Source: CAD feature listing. Evaluate the final solid. Frame: model axes, mm. A direction names the side the tool comes from. Round coordinates to 2 decimals unless told otherwise and drop trailing zeros. Loops run counter-clockwise (first coordinate to the right, second up) from the corner with the lowest first, then second, coordinate; pieces in that order, holes last. Notation, with made-up numbers: M 55.25,89.5 L 98.25,89.5 A26 ccw 98.25,111.5 Z; hole C 70,81.25 d9. An arc over 180 degrees is marked long. One line per item, written item: value.
from build123d import *

# Parameters (mm, degrees)
SKETCH1_R                      = 1.27
SKETCH1_R_2                    = 3.81
BOSS_EXTRUDE1_DEPTH            = 5.08
F_15_0_18_DIAMETER_HOLE1_D     = 4.572
SKETCH5_W                      = 15.24
SKETCH5_H                      = 3.81
CUT_EXTRUDE1_DEPTH             = 5.08
FILLET1_R                      = 1.27
CUT_EXTRUDE3_START             = 5.334
SKETCH8_R                      = 1.651
CUT_EXTRUDE3_DEPTH             = 0.762
SCALE1_SCALE                   = 1.5
F_35_0_11_DIAMETER_HOLE1_D     = 2.794
F_35_0_11_DIAMETER_HOLE1_DEPTH = 6.35
F_35_0_11_DIAMETER_HOLE1_TIP   = 0.839402285


with BuildPart() as part:
    # Sketch1 → Boss-Extrude1 (new, symmetric)
    with BuildSketch(Plane.XY):
        with BuildLine():
            Line((-20.909409051, -2.54), (-4.399409051, -2.54))
            ThreePointArc((-4.399409051, -2.54), (5.08, 0), (-4.399409051, 2.54))
            Line((-4.399409051, 2.54), (-20.909409051, 2.54))
            ThreePointArc((-20.909409051, 2.54), (-23.449409051, 0), (-20.909409051, -2.54))
        make_face()
        with Locations((-20.909409051, 0)):
            Circle(SKETCH1_R, mode=Mode.SUBTRACT)
        Circle(SKETCH1_R_2, mode=Mode.SUBTRACT)
    extrude(amount=BOSS_EXTRUDE1_DEPTH, both=True)

    # #15 (0.18) Diameter Hole1 (through all)
    with Locations(Plane(origin=(0, 2.54, 0), x_dir=(1, 0, 0), z_dir=(0, 1, 0))):
        with Locations((-12.019409051, 0)):
            Hole(F_15_0_18_DIAMETER_HOLE1_D / 2)

    # Sketch5 → Cut-Extrude1 (cut)
    with BuildSketch(Plane(origin=(0, 2.54, 0), x_dir=(1, 0, 0), z_dir=(0, 1, 0))):
        with Locations((-23.449409051, 0)):
            Rectangle(SKETCH5_W, SKETCH5_H)
    extrude(amount=-CUT_EXTRUDE1_DEPTH, mode=Mode.SUBTRACT)

    # Fillet1
    fillet1_edges = [part.edges().sort_by_distance(p)[0] for p in [
        (-15.829409051, 0, 1.905),
        (-15.829409051, 0, -1.905),
    ]]
    fillet(fillet1_edges, radius=FILLET1_R)

    # Sketch8 → Cut-Extrude3 (cut)
    with BuildSketch(Plane(origin=(0, 0, 0), x_dir=(0, 0, -1), z_dir=(1, 0, 0)).offset(CUT_EXTRUDE3_START)):
        Circle(SKETCH8_R)
    extrude(amount=-CUT_EXTRUDE3_DEPTH, mode=Mode.SUBTRACT)


with BuildPart() as part_1:
    # Scale1: scaled about (-8.355295552, 4.7607e-05, -6.308e-06)
    add(part.part.scale(SCALE1_SCALE).moved(Location((4.177647776, -2.3804e-05, 3.154e-06))))

    # #35 (0.11) Diameter Hole1
    with Locations(Plane(origin=(11.035535864, 0, 0), x_dir=(0, 0, -1), z_dir=(1, 0, 0))):
        with Locations((0, 0)):
            Hole(F_35_0_11_DIAMETER_HOLE1_D / 2, depth=F_35_0_11_DIAMETER_HOLE1_DEPTH)
            with Locations((0, 0, -(F_35_0_11_DIAMETER_HOLE1_DEPTH + F_35_0_11_DIAMETER_HOLE1_TIP / 2))):  # 118° drill point
                Cone(0, F_35_0_11_DIAMETER_HOLE1_D / 2, F_35_0_11_DIAMETER_HOLE1_TIP, mode=Mode.SUBTRACT)


solid = part_1.part
1. Reachability of faces 1 (the face through (-14.6, 3.81, 3.5)), 2 (the face through (11.3, 1.7, 1.8)), 3 (the face through (-20.139, -0.053, -2.314)) from +Z, -Z, +X, -X, +Y, -Y: full face, straight path, thin tool, end or side. Return the list, or none.
Report:
face 1: +Z, -Z, -X, +Y
face 2: +X
face 3: -X, +Y, -Y
2. Pull-direction query (X, two-part tool) for faces 4 (the face through (10.693, 3.951, 0.107)), 5 (the face through (-10, 0, -7.62)), 6 (the face through (-10.426, -0.053, -0.151)), 7 (the face through (-30.996, 0.084, 5.272)); classes: released by +X, released by -X, zero draft, split by the parting line, or undercut.
Report:
face 4: split by the parting line
face 5: zero draft
face 6: undercut
face 7: released by -X
3. Section query A-A (z = 0.5). Return the cut outline in (x, y) (3 decimals).
Report:
outline: M -19.566,-3.81 L -17.244,-3.81 L -17.244,3.81 L -19.566,3.81 Z; M -10.459,-3.81 L -2.421,-3.81 A7.62 ccw 11.401,-2.426 L 11.036,-2.426 L 11.036,-1.304 L 9.742,-1.304 A5.715 cw long 9.742,1.304 L 11.036,1.304 L 11.036,2.425 L 11.401,2.425 A7.62 ccw -2.421,3.81 L -10.459,3.81 Z
4. Ray query, line 1 (X direction, y = -1, z = -3); line 2 (X direction, y = -0.75, z = 3.5); line 3 (X direction, y = -1.5, z = -4.75). Return the intervals inside material, ascending. Write a range as [from, to].
Report:
line 1: x = [-30.86, -28.81], [-25.57, -15.51], [-12.19, -1.45], [9.8, 11.73]
line 2: x = [-30.92, -28.94], [-25.44, -1.49], [9.84, 11.76]
line 3: x = [-30.69, -28.36], [-26.01, -1.34], [9.69, 11.65]
5. Section query D-D (x = -6.5). Return the cut outline in (y, z), and give its area (3 significant figures).
Report:
outline: M -3.81,-7.62 L 3.81,-7.62 L 3.81,7.62 L -3.81,7.62 Z
area: 116 mm2
6. Pin query (flat end, axial travel): pin 1 (2.5 mm diameter, centred on x = -26.5, y = 0.5, fed in from -Z); pin 2 (7.5 mm diameter, centred on x = -9, z = 1.5, fed in from -Y); pin 3 (3 mm diameter, centred on y = 0, z = 0, fed in from -X); pin 4 (2.5 mm diameter, centred on y = -0.5, z = 0.5, fed in from +X). Return the tip coordinate at first contact, or that it passes through.
Report:
pin 1: stops at z = -7.62
pin 2: stops at y = -3.81
pin 3: stops at x = -19.65
pin 4: stops at x = 11.04
7. Section query C-C (z = -6). Return the cut outline in (x, y) (3 decimals), and give its area (3 significant figures).
Report:
outline: M -27.186,-3.81 L -2.421,-3.81 A7.62 ccw long -2.421,3.81 L -27.186,3.81 A3.81 ccw Z; hole C -27.186,0 d3.81; hole C 4.178,0 d11.43
area: 275 mm2
8. Section query B-B (x = 8). Return the cut outline in (y, z), and give its area (3 significant figures).
Report:
outline: M -6.59,-7.62 L -4.25,-7.62 L -4.25,7.62 L -6.59,7.62 Z; M 4.25,-7.62 L 6.59,-7.62 L 6.59,7.62 L 4.25,7.62 Z
area: 71.4 mm2
